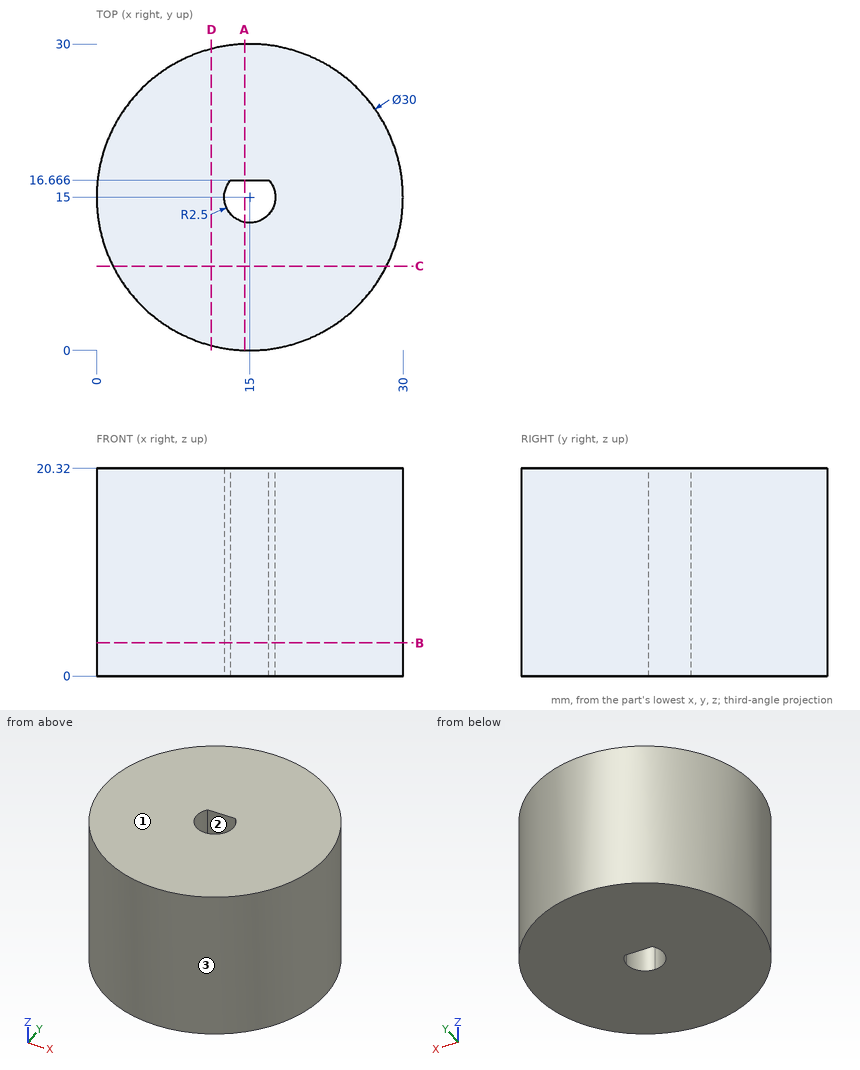
Part print with two shaded views. Sizes in mm from the minimum x, y, z corner. Round coordinates to 2 decimals unless told otherwise and drop trailing zeros. Order: outer loops, then holes, each group sorted by start corner. A loop starts at its lowest first (then second) coordinate and runs counter-clockwise, first axis right, second up. Notation, with made-up numbers: M 84.5,-21 L 127.5,-21 A33 ccw 127.5,11 Z; hole C 13,75 d8. An arc over 180 degrees is marked long. Put each result on its own line as item: value. Start each with the question number.
1. Slice it at A-A on x = 14.5. List the corners of the cut face in (y, z).
2. Drop flat-ended pins along their axis: pin 1 (1.5 mm diameter, centred on y = 3.5, z = 6.5, fed in from -X); pin 2 (6 mm diameter, centred on x = 8.5, z = 16, fed in from -Y); pin 3 (10 mm diameter, centred on y = 9.5, z = 12.5, fed in from -X). Give the stop position or say it passes through.
3. Two-plate mould, pull along Y, no slides. Class the marked faces 1, 2 and 3: +Y half, -Y half, draft (parallel to the pull), parting line (faces both ways), or undercut.
4. Slice it at C-C on y = 8.25. List the corners of the cut face in (x, z) (1 decimal).
5. Slice it at D-D on x = 11.25. List the corners of the cut face in (y, z), then the cut area to 3 significant figures.
6. Drill centre lines: probe 1 along Y at (x, z) = (13.75, 17.5) (1 decimal); probe 2 along Y at (x, z) = (14.75, 7.5); probe 3 along Y at (x, z) = (19.25, 5) (1 decimal). Where is each one in solid material? Low to high. Write a range as [from, to].
7. Slice it at B-B on z = 3.25. List the corners of the cut face in (x, y).
Findings:
1. outline: M 0.01,0 L 12.55,0 L 12.55,20.32 L 0.01,20.32 Z; M 16.67,0 L 29.99,0 L 29.99,20.32 L 16.67,20.32 Z
2. pin 1: x = 4.54
2. pin 2: y = 0.41
2. pin 3: x = 0.01
3. face 1: draft
3. face 2: undercut
3. face 3: parting line
4. outline: M 1.6,0 L 28.4,0 L 28.4,20.3 L 1.6,20.3 Z
5. outline: M 0.48,0 L 29.52,0 L 29.52,20.32 L 0.48,20.32 Z
5. area: 590 mm2
6. probe 1: [0.1, 12.8], [16.7, 29.9]
6. probe 2: [0, 12.51], [16.67, 30]
6. probe 3: [0.6, 29.4]
7. outline: C 15,15 d30; hole M 13.14,16.67 A2.5 ccw long 17.5,15 A2.5 ccw 16.86,16.67 Z
